Build history of the part. All positions in model axes, mm. Face numbers are marked on the shaded views. Round coordinates to 2 decimals unless told otherwise and drop trailing zeros. Loops run counter-clockwise (first coordinate to the right, second up) from the corner with the lowest first, then second, coordinate; pieces in that order, holes last. Notation, with made-up numbers: M 44.5,45.5 L 57.5,45.5 A28 ccw 57.5,63.5 Z; hole C 54,59 d1. An arc over 180 degrees is marked long. Use one line per item in the form item = value. Start each with the question number.
```python
from build123d import *

# Parameters (mm, degrees)
SKETCH1_W                    = 38.421818
SKETCH1_H                    = 25.4
BOSS_EXTRUDE1_DEPTH          = 298.45
F_3_8_16_TAPPED_HOLE1_D      = 7.9375
F_3_8_0_375_DIAMETER_HOLE2_D = 9.525
SKETCH11_W                   = 53.975
SKETCH11_H                   = 38.421818
CUT_EXTRUDE2_DEPTH           = 12.7


with BuildPart() as part:
    # Sketch1 → Boss-Extrude1 (new body)
    with BuildSketch(Plane(origin=(0, 0, 0), x_dir=(0, 0, -1), z_dir=(1, 0, 0))):
        with Locations((19.210909, 12.7)):
            Rectangle(SKETCH1_W, SKETCH1_H)
    extrude(amount=BOSS_EXTRUDE1_DEPTH)

    # 3/8-16 Tapped Hole1 (through all)
    with Locations(Plane(origin=(0, 0, -38.421818), x_dir=(-1, 0, 0), z_dir=(0, 0, -1))):
        with Locations((-284.1625, 12.7), (-14.2875, 12.7)):
            Hole(F_3_8_16_TAPPED_HOLE1_D / 2)

    # 3/8 (0.375) Diameter Hole2 (through all)
    with Locations(Plane(origin=(0, 25.4, 0), x_dir=(1, 0, 0), z_dir=(0, 1, 0))):
        with Locations((30.4121566, 12.7), (274.3878434, 12.7)):
            Hole(F_3_8_0_375_DIAMETER_HOLE2_D / 2)

    # Sketch11 → Cut-Extrude2 (cut)
    with BuildSketch(Plane.XZ):
        with Locations((149.225, -19.210909)):
            Rectangle(SKETCH11_W, SKETCH11_H)
    extrude(amount=-CUT_EXTRUDE2_DEPTH, mode=Mode.SUBTRACT)


solid = part.part
```
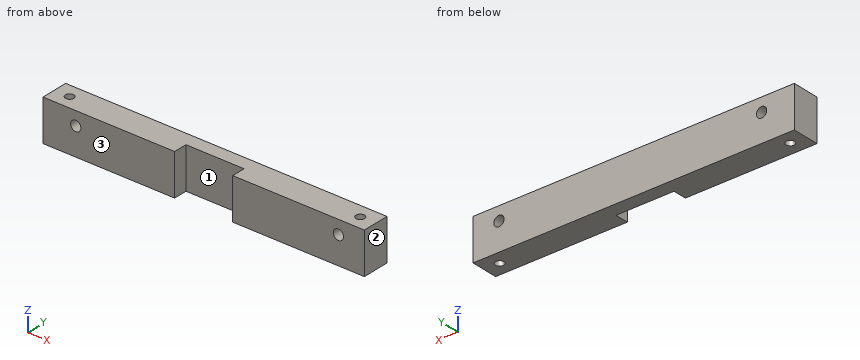
Q1. Saw through at B-B (z = -34.5). Give the cut face in (x, y).
Q2. Pull direction X, two halves, no side cores. Call the marked faces 1, 2 and 3: pulls with the +X half, pulls with the -X half, needs draft (parallel to the pull), parting line crosses it, or undercut.
Q3. Saw through at A-A (z = -12.7). Give the cut face in (x, y), and give its area (3 significant figures).
Q4. Wall check: probe 1 along X at (y, z) = (7, -19); probe 2 along Z at (x, y) = (270.5, 2); probe 3 along Y at (x, z) = (129, -12). Give the ranges that are in metal, low to high.
Q5. Drop flat-ended pins along their axis: P1, Ø3, axis at y = 19.5, z = -11.5, coming from the -X side; P2, Ø5.5, axis at x = 30.41, z = -12.7, coming from the +Y side. Give the stop position or say it passes through.
Filled in:
q1.outline = M 0,0 L 122.24,0 L 122.24,12.7 L 176.21,12.7 L 176.21,0 L 298.45,0 L 298.45,25.4 L 0,25.4 Z; hole C 14.29,12.7 d7.94; hole C 284.16,12.7 d7.94
q2.face_1 = undercut
q2.face_2 = pulls with the +X half
q2.face_3 = needs draft
q3.outline = M 0,0 L 25.65,0 L 25.65,25.4 L 0,25.4 Z; M 35.17,0 L 122.24,0 L 122.24,12.7 L 176.21,12.7 L 176.21,0 L 269.63,0 L 269.63,25.4 L 35.17,25.4 Z; M 279.15,0 L 298.45,0 L 298.45,25.4 L 279.15,25.4 Z; hole C 14.29,12.7 d7.94; hole C 284.16,12.7 d7.94
q3.area = 6,310 mm²
q4.probe_1 = 0 to 122.24, 176.21 to 298.45
q4.probe_2 = -38.42 to -15.45, -9.95 to 0
q4.probe_3 = 12.7 to 25.4
q5.P1 = 0
q5.P2 = through
